Could you check a few things on this model? Use its own coordinates, in mm. A direction names the side the tool comes from. Round coordinates to 2 decimals unless told otherwise and drop trailing zeros. Order: outer loops, then holes, each group sorted by start corner. A loop starts at its lowest first (then second) coordinate and runs counter-clockwise, first axis right, second up. Notation, with made-up numbers: M 42,-7.75 L 86,-7.75 A33 cw 86,28.25 Z; hole C 68,-12.5 d4. An arc over 180 degrees is marked long. Write each question's results on one line, items separated by ' | '. Start each with the question number.
1. Suppose I cut it at A-A on x = 0. Write out the boundary of the cut face in (y, z), and give its area (3 significant figures).
2. We'd pull the mould along X, two halves only. Please class faces 5 (the cylindrical face through (20.765, -39.923, 2.986)), 6 (the cylindrical face through (-0.712, 33.154, 2.958)), 7 (the flat face through (9, -9, 0)): released by +X, released by -X, zero draft, split by the parting line, or undercut.
3. Suppose I cut it at B-B on z = 1. Write out the boundary of the cut face in (x, y), and give its area (3 significant figures).
4. Suppose I cut it at C-C on y = -7. Give the number of separate pieces and of enclosed holes in the cut face, and give its area (3 significant figures).
5. For faces 1 (the flat face through (24, -3.248, 3)), 2 (the flat face through (9, -9, 6)), 3 (the cylindrical face through (23.217, 2.677, 5.399)), 4 (the cylindrical face through (23.491, -2.677, 0.601)), which set-ups out of +Z, -Z, +X, -X, +Y, -Y let a thin tool reach every point of the face, with its end or its side?
6. Please list where these lines run through material, in increasing order: L1, parallel to Y at x = 16, z = 4.5; L2, parallel to Y at x = 4, z = 3.25; L3, parallel to X at y = -8, z = 2.
7. I'm going to push flat-ended pins straight in: pin 1 (1 mm diameter, centred on x = 20.5, z = 3, fed in from -Y); pin 2 (0.6 mm diameter, centred on x = 26, z = 2.5, fed in from +Y); pin 3 (2 mm diameter, centred on x = -28, z = 3, fed in from +Y); pin 4 (8 mm diameter, centred on x = 2, y = 20, fed in from -Z). Where does each tip first touch, or does it pass through?
from build123d import *

# Parameters (mm, degrees)
F0_R     = 45
F1_DEPTH = 6
F2_R     = 2


with BuildPart() as f1:
    # F0 (on Top) → F1 (new body)
    with BuildSketch(Plane.XY):
        Circle(F0_R)
        with BuildLine():
            ThreePointArc((33.0021725985, 3.2475610053), (33.1217003385, 1.6257353391), (33.1615748828, 0))
            ThreePointArc((33.1615748828, 0), (33.1217003385, -1.6257353391), (33.0021725985, -3.2475610053))
            ThreePointArc((33.0021725985, -3.2475610053), (0, -33.1615748828), (-33.0021725985, -3.2475610053))
            ThreePointArc((-33.0021725985, -3.2475610053), (-33.1615748828, 0), (-33.0021725985, 3.2475610053))
            ThreePointArc((-33.0021725985, 3.2475610053), (0, 33.1615748828), (33.0021725985, 3.2475610053))
        make_face(mode=Mode.SUBTRACT)
        with BuildLine():
            Line((-15.2860053166, 3.2475610053), (-33.0021725985, 3.2475610053))
            ThreePointArc((-33.0021725985, 3.2475610053), (-33.1615748828, 0), (-33.0021725985, -3.2475610053))
            Line((-33.0021725985, -3.2475610053), (-15.2860053166, -3.2475610053))
            ThreePointArc((-15.2860053166, -3.2475610053), (-15.6271754013, 0), (-15.2860053166, 3.2475610053))
        make_face()
        with BuildLine():
            Line((-10.7188314436, 3.2475610053), (-15.2860053166, 3.2475610053))
            ThreePointArc((-15.2860053166, 3.2475610053), (-15.6271754013, 0), (-15.2860053166, -3.2475610053))
            Line((-15.2860053166, -3.2475610053), (-10.7188314436, -3.2475610053))
            ThreePointArc((-10.7188314436, -3.2475610053), (-11.2, 0), (-10.7188314436, 3.2475610053))
        make_face()
        with BuildLine():
            Line((10.7188314436, 3.2475610053), (15.2860053166, 3.2475610053))
            ThreePointArc((15.2860053166, 3.2475610053), (0, 15.6271754013), (-15.2860053166, 3.2475610053))
            Line((-15.2860053166, 3.2475610053), (-10.7188314436, 3.2475610053))
            ThreePointArc((-10.7188314436, 3.2475610053), (0, 11.2), (10.7188314436, 3.2475610053))
        make_face()
        with BuildLine():
            ThreePointArc((-15.2860053166, -3.2475610053), (0, -15.6271754013), (15.2860053166, -3.2475610053))
            Line((15.2860053166, -3.2475610053), (10.7188314436, -3.2475610053))
            ThreePointArc((10.7188314436, -3.2475610053), (0, -11.2), (-10.7188314436, -3.2475610053))
            Line((-10.7188314436, -3.2475610053), (-15.2860053166, -3.2475610053))
        make_face()
        with BuildLine():
            ThreePointArc((15.6271754013, 0), (15.5416488393, 1.6327162575), (15.2860053166, 3.2475610053))
            Line((15.2860053166, 3.2475610053), (10.7188314436, 3.2475610053))
            ThreePointArc((10.7188314436, 3.2475610053), (11.0790548371, 1.6415065993), (11.2, 0))
            ThreePointArc((11.2, 0), (11.0790548371, -1.6415065993), (10.7188314436, -3.2475610053))
            Line((10.7188314436, -3.2475610053), (15.2860053166, -3.2475610053))
            ThreePointArc((15.2860053166, -3.2475610053), (15.5416488393, -1.6327162575), (15.6271754013, 0))
        make_face()
        with BuildLine():
            ThreePointArc((33.0021725985, -3.2475610053), (33.1217003385, -1.6257353391), (33.1615748828, 0))
            ThreePointArc((33.1615748828, 0), (33.1217003385, 1.6257353391), (33.0021725985, 3.2475610053))
            Line((33.0021725985, 3.2475610053), (15.2860053166, 3.2475610053))
            ThreePointArc((15.2860053166, 3.2475610053), (15.5416488393, 1.6327162575), (15.6271754013, 0))
            ThreePointArc((15.6271754013, 0), (15.5416488393, -1.6327162575), (15.2860053166, -3.2475610053))
            Line((15.2860053166, -3.2475610053), (33.0021725985, -3.2475610053))
        make_face()
    extrude(amount=F1_DEPTH)

    # F2
    f2_edges = [f1.edges().sort_by_distance(p)[0] for p in [
        (-45, 0, 6),
        (-24.144089, -3.247561, 6),
        (0, -15.627175, 0),
        (24.144089, -3.247561, 6),
        (0, 15.627175, 6),
        (-24.144089, 3.247561, 6),
        (24.144089, 3.247561, 6),
        (-45, 0, 0),
        (0, 15.627175, 0),
        (24.144089, 3.247561, 0),
        (0, -15.627175, 6),
        (-24.144089, 3.247561, 0),
        (-24.144089, -3.247561, 0),
        (24.144089, -3.247561, 0),
    ]]
    fillet(f2_edges, radius=F2_R)


solid = f1.part
Filled sheet:
1) outline: M -45,2 A2 ccw -43,0 L -33.16,0 L -33.16,6 L -43,6 A2 ccw -45,4 Z; M -15.63,2 A2 ccw -13.63,0 L -11.2,0 L -11.2,6 L -13.63,6 A2 ccw -15.63,4 Z; M 11.2,0 L 13.63,0 A2 ccw 15.63,2 L 15.63,4 A2 ccw 13.63,6 L 11.2,6 Z; M 33.16,0 L 43,0 A2 ccw 45,2 L 45,4 A2 ccw 43,6 L 33.16,6 Z | area: 188 mm^2
2) face 5: split by the parting line | face 6: undercut | face 7: zero draft
3) outline: C 0,0 d89.46; hole M -33.03,-2.98 A33.16 ccw 33.03,-2.98 L 15.07,-2.98 A15.36 cw -15.07,-2.98 Z; hole M -33.03,2.98 L -15.07,2.98 A15.36 cw 15.07,2.98 L 33.03,2.98 A33.16 ccw Z; hole C 0,0 d22.4 | area: 3,390 mm^2
4) separate pieces: 4 | enclosed holes: 0 | area: 200 mm^2
5) face 1: +Z, -Z | face 2: +Z, +X, -X, +Y, -Y | face 3: +Z | face 4: -Z
6) L1: y = -41.99 to -29.05, -3.18 to 3.18, 29.05 to 41.99 | L2: y = -44.82 to -32.92, -15.11 to -10.46, 10.46 to 15.11, 32.92 to 44.82 | L3: x = -44.28 to -32.18, -13.42 to -7.84, 7.84 to 13.42, 32.18 to 44.28
7) pin 1: stops at y = -40.31 | pin 2: stops at y = 36.94 | pin 3: stops at y = 36 | pin 4: passes through
